Build history of the part. All positions in model axes, mm. A direction names the side the tool comes from. Coordinates: 2 decimals unless noted, no trailing zeros. Loops run counter-clockwise (first coordinate to the right, second up) from the corner with the lowest first, then second, coordinate; pieces in that order, holes last. Notation, with made-up numbers: (-29.75, 2.25) -> (24.25, 2.25) arc R21 cw to (24.25, 15.25) -> close; hole circle Ø6 at (-8, 39.25). An arc over 180 degrees is marked (long way). One line per item, written item: value. Start each with the question number.
```python
from build123d import *

# Parameters (mm, degrees)
SKETCH2_W          = 8.307416394
SKETCH2_H          = 3.81
SKETCH2_W_2        = 3.81
SKETCH2_H_2        = 8.307416394
CUT_EXTRUDE1_DEPTH = 0.889
CUT_EXTRUDE2_DEPTH = 1.778


with BuildPart() as part:
    # Sketch1 → Revolve1 (revolve)
    with BuildSketch(Plane.XY, mode=Mode.PRIVATE) as revolve1_sk:
        Polygon((5.08, 14.859), (6.985, 14.859), (6.985, 5.334), (11.303, 5.334), (14.097, 7.9375), (17.907, 7.9375), (17.907, 6.1595), (15.6845, 6.1595), (15.6845, 3.81), (17.907, 3.81), (17.907, 0), (16.002, 0), (16.002, 3.039995698), (11.198857665, 3.039995698), (12.954, 0), (8.9535, 0), (8.9535, -0.889), (4.8895, -0.889), (4.8895, 0), (1.524, 0), (1.524, 5.715), (5.08, 5.715), align=None)
    revolve(revolve1_sk.sketch.rotate(Axis((0, 0, 0), (0, 1, 0)), 90), axis=Axis((0, 0, 0), (0, 1, 0)))

    # Sketch2 → Cut-Extrude1 (cut)
    with BuildSketch(Plane(origin=(0, -0.889, 0), x_dir=(-1, 0, 0), z_dir=(0, 1, 0))):
        with Locations((6.058708197, 0)):
            Rectangle(SKETCH2_W, SKETCH2_H)
        with Locations((0, 6.058708197)):
            Rectangle(SKETCH2_W_2, SKETCH2_H_2)
        with Locations((0, -6.058708197)):
            Rectangle(SKETCH2_W_2, SKETCH2_H_2)
        with Locations((-6.058708197, 0)):
            Rectangle(SKETCH2_W, SKETCH2_H)
    extrude(amount=CUT_EXTRUDE1_DEPTH, mode=Mode.SUBTRACT)

    # Sketch2_3 → Cut-Extrude2 (cut)
    with BuildSketch(Plane(origin=(0, -0.889, 0), x_dir=(-1, 0, 0), z_dir=(0, 1, 0))):
        with BuildLine():
            Line((-12.638378045, 0.188485038), (-12.96898322, 0.813026828))
            ThreePointArc((-12.96898322, 0.813026828), (-12.992820329, 0.205324805), (-12.988197288, -0.402826973))
            ThreePointArc((-12.988197288, -0.402826973), (-12.64770122, -0.205131646), (-12.638378045, 0.188485038))
        make_face()
        with BuildLine():
            Line((-0.188485038, -12.638378045), (-0.813026828, -12.96898322))
            ThreePointArc((-0.813026828, -12.96898322), (-0.205324805, -12.992820329), (0.402826973, -12.988197288))
            ThreePointArc((0.402826973, -12.988197288), (0.205131646, -12.64770122), (-0.188485038, -12.638378045))
        make_face()
        with BuildLine():
            Line((12.638378045, -0.188485038), (12.96898322, -0.813026828))
            ThreePointArc((12.96898322, -0.813026828), (12.992820329, -0.205324805), (12.988197288, 0.402826973))
            ThreePointArc((12.988197288, 0.402826973), (12.64770122, 0.205131646), (12.638378045, -0.188485038))
        make_face()
        with BuildLine():
            ThreePointArc((-0.402826973, 12.988197288), (-0.205131646, 12.64770122), (0.188485038, 12.638378045))
            Line((0.188485038, 12.638378045), (0.813026828, 12.96898322))
            ThreePointArc((0.813026828, 12.96898322), (0.205324805, 12.992820329), (-0.402826973, 12.988197288))
        make_face()
    extrude(amount=CUT_EXTRUDE2_DEPTH, mode=Mode.SUBTRACT)


solid = part.part
```
Item 1: Two-plate mould, pull along X, no slides. Class faces 6 (the face through (5, -0.889, -5)), 7 (the face through (-6.38, -0.45, 6.28)), 8 (the face through (-3.397, 2.85, -10.786)): +X half, -X half, draft (parallel to the pull), parting line (faces both ways), or undercut.
Item 2: Drop flat-ended pins along their axis: pin 1 Ø11.5 at (x, z) = (4.5, 1.5) entering from +Y; pin 2 Ø5 at (x, z) = (12, 4.5) entering from +Y; pin 3 Ø1 at (x, y) = (2.5, 7) entering from -Z; pin 4 Ø5 at (x, y) = (-7, 5.5) entering from -Z. Give the stop position or say it passes through.
Item 3: Tool access for faces 1 (the face through (6.38, -0.45, -6.28)), 2 (the face through (-6.28, -0.45, -6.38)), 3 (the face through (-3.439, -0.438, -3.476)), 4 (the face through (6.7, -0.5, -1.905)), 5 (the face through (4.9, 5.334, -5.2)): list every direction of +Z, -Z, +X, -X, +Y, -Y with a clear straight run to the whole face (end or side of a thin tool).
Item 4: Band-saw the part on A-A, the plane y = 2.5. List the corners of the cut face in (x, z), and give its area (3 significant figures).
Item 5: Probe probe 1 along X at (y, z) = (3.3, 0); probe 2 along X at (y, z) = (2.15, 0); probe 3 along X at (y, z) = (12.25, 0) (3 decimals). List the from-to ranges inside material, lowest first.
Worked out:
1. face 6: draft
1. face 7: -X half
1. face 8: undercut
2. pin 1: stops at y = 14.86
2. pin 2: stops at y = 7.94
2. pin 3: stops at z = -17.79
2. pin 4: stops at z = -17.31
3. face 1: -Z, +X, -Y
3. face 2: -Z, -X, -Y
3. face 3: -Y
3. face 4: +X, -X, -Y
3. face 5: +Y
4. outline: circle Ø35.81 at (0, 0); circle Ø23.02 at (0, 0); hole circle Ø32 at (0, 0); hole circle Ø3.05 at (0, 0)
4. area: 612 mm²
5. probe 1: x = -17.91 to -1.52, 1.52 to 17.91
5. probe 2: x = -17.91 to -16, -11.71 to -1.52, 1.52 to 11.71, 16 to 17.91
5. probe 3: x = -6.985 to -5.08, 5.08 to 6.985
